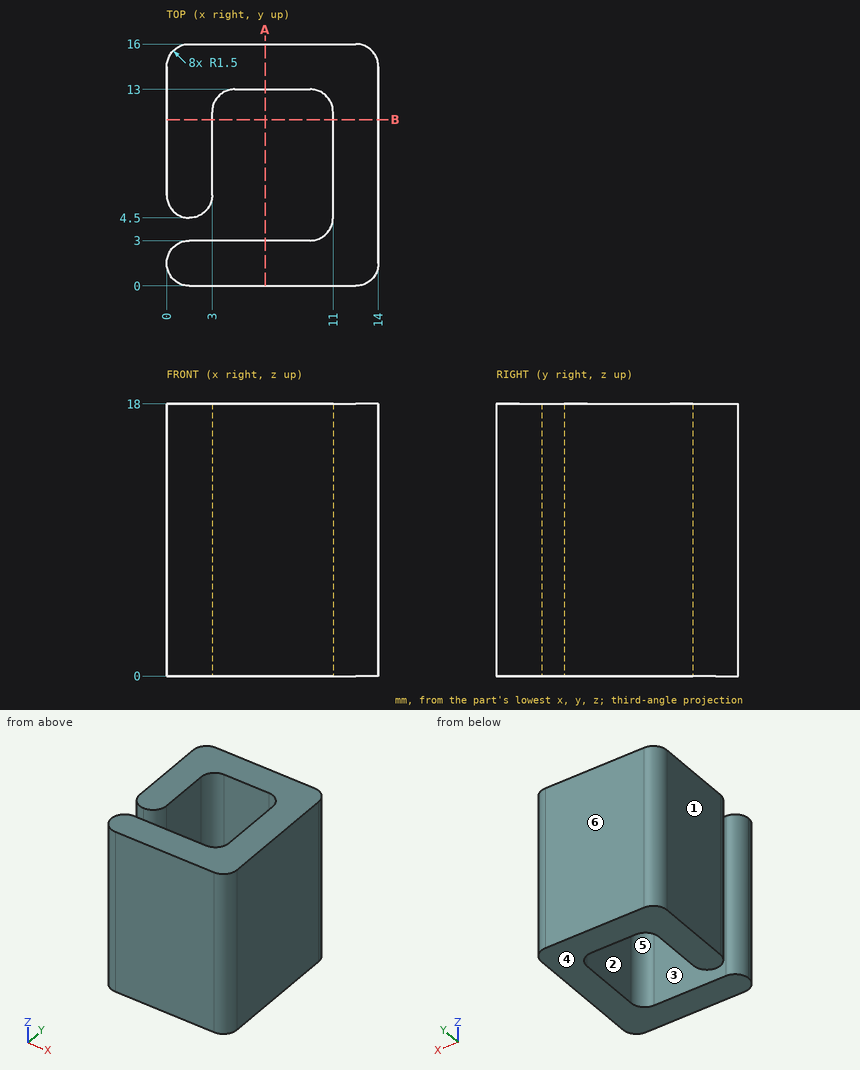
Geometry: see drawing. Coordinates: mm, zero at the bounding-box minimum. A direction names the side the tool comes from. Round coordinates to 2 decimals unless told otherwise and drop trailing zeros. Write each loop counter-clockwise with the first axis right and the second up, starting at its lowest first coordinate (ties: lowest second). Pieces come first, ordered by that corner, then holes. Notation, with made-up numbers: M 49,-27 L 62,-27 A22 ccw 62,-4 Z; hole C -9.5,-28.75 d4. An arc over 180 degrees is marked long. Answer as a JSON object with one key per item and string values. Group by question number.
(1) Section query B-B on y = 11. Output: boundary loops of the cut face in (x, z), then the cut area to 3 significant figures.
(2) Ray query, line 1 (Y direction, x = 4.5, z = 1.5); line 2 (X direction, y = 9.5, z = 3); line 3 (X direction, y = 5, z = 10.75). Return the intervals inside material, ascending. Write a range as [from, to].
(3) Section query A-A on x = 6.5. Output: boundary loops of the cut face in (y, z).
(4) Mould query, pull axis Y, two halves, no side actions, for the marked faces 4, 5 and 6. Classes: +Y half, -Y half, draft (parallel to the pull), parting line (faces both ways), or undercut.
(5) First-contact query: pin 1 (3.5 mm diameter, centred on y = 9, z = 10.5, fed in from -X); pin 2 (6 mm diameter, centred on x = 7.5, y = 8.5, fed in from -Z). Flat tips, straight axial feed; report the tip coordinate or a pass-through.
(6) Reachability of the marked faces 1, 2 and 3 from +Z, -Z, +X, -X, +Y, -Y: full face, straight path, thin tool, end or side. Return the list, or none.
Computed values:
{
 "1": {"outline": "M 0,0 L 3,0 L 3,18 L 0,18 Z; M 11,0 L 14,0 L 14,18 L 11,18 Z", "area": "108 mm^2"},
 "2": {"line 1": "[0, 3], [13, 16]", "line 2": "[0, 3], [11, 14]", "line 3": "[0.38, 2.62], [11, 14]"},
 "3": {"outline": "M 0,0 L 3,0 L 3,18 L 0,18 Z; M 13,0 L 16,0 L 16,18 L 13,18 Z"},
 "4": {"face 4": "draft", "face 5": "undercut", "face 6": "+Y half"},
 "5": {"pin 1": "x = 0", "pin 2": "through"},
 "6": {"face 1": "+Z, -Z, -X, +Y, -Y", "face 2": "+Z, -Z", "face 3": "+Z, -Z, -X"}
}
